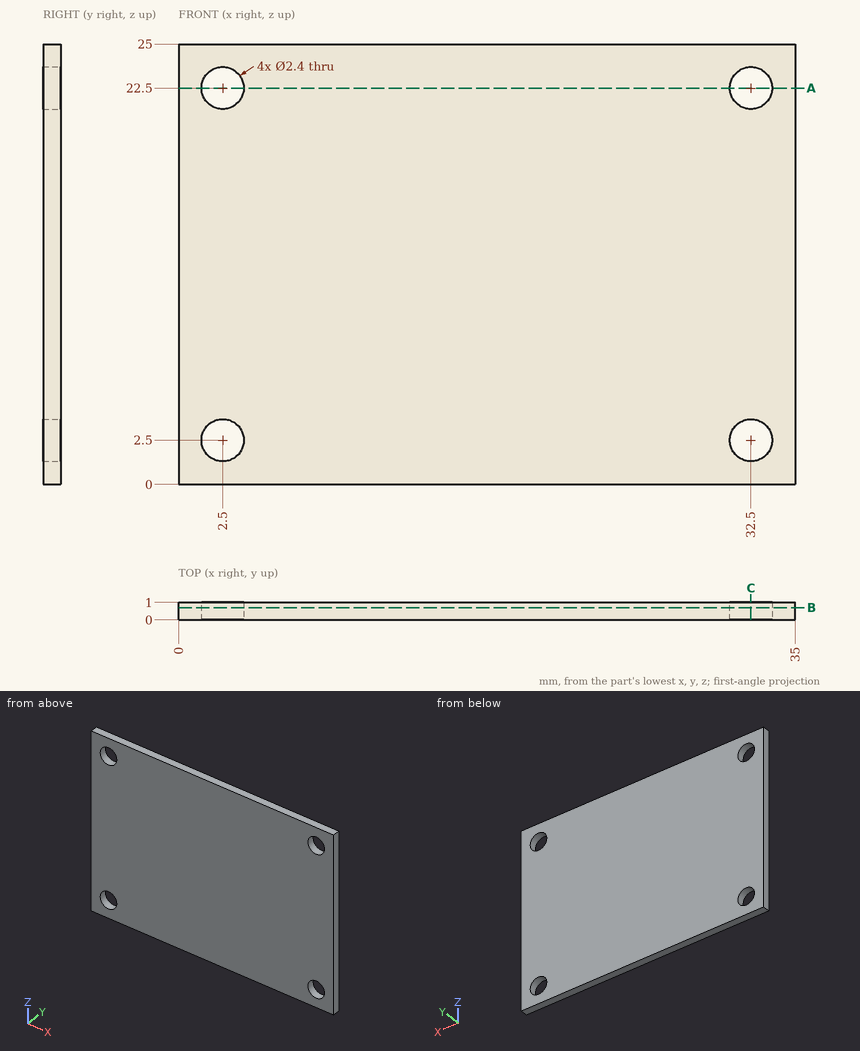
Here's the drawing with two shaded views (mm, measured from the low corner). I have some questions. Give positions to 0.01 mm unless a question says otherwise; leave off trailing zeros. Write each loop counter-clockwise with the first axis right and the second up, starting at its lowest first coordinate (ties: lowest second). Pieces come first, ordered by that corner, then holes. Notation, with made-up numbers: (18.5, 40) -> (59.5, 40) arc R19 cw to (59.5, 75) -> close; hole circle Ø9 at (46, 81). An arc over 180 degrees is marked (long way). One line per item, written item: value.
Q1. Imagine slicing it at C-C on x = 32.5. Please give me the cut outline in (y, z).
Results found:
outline: (0, 0) -> (1, 0) -> (1, 1.3) -> (0, 1.3) -> close; (0, 3.7) -> (1, 3.7) -> (1, 21.3) -> (0, 21.3) -> close; (0, 23.7) -> (1, 23.7) -> (1, 25) -> (0, 25) -> close
Q2. Imagine slicing it at A-A on z = 22.5. Please give me the cut outline in (x, y).
Results found:
outline: (0, 0) -> (1.3, 0) -> (1.3, 1) -> (0, 1) -> close; (3.7, 0) -> (31.3, 0) -> (31.3, 1) -> (3.7, 1) -> close; (33.7, 0) -> (35, 0) -> (35, 1) -> (33.7, 1) -> close
Q3. Please list where these lines run through material, in increasing order: line 1 (X direction, y = 0.2, z = 2.5); line 2 (Z direction, x = 2.5, y = 0.7); line 3 (Z direction, x = 32, y = 0.8). Write a range as [from, to].
Results found:
line 1: x = [0, 1.3], [3.7, 31.3], [33.7, 35]
line 2: z = [0, 1.3], [3.7, 21.3], [23.7, 25]
line 3: z = [0, 1.41], [3.59, 21.41], [23.59, 25]
Q4. Imagine slicing it at B-B on y = 0.7. Please give me the cut outline in (x, z), and give its area (3 significant figures).
Results found:
outline: (0, 0) -> (35, 0) -> (35, 25) -> (0, 25) -> close; hole circle Ø2.4 at (2.5, 2.5); hole circle Ø2.4 at (2.5, 22.5); hole circle Ø2.4 at (32.5, 2.5); hole circle Ø2.4 at (32.5, 22.5)
area: 857 mm^2
